Source: CAD feature listing. Evaluate the final solid. Frame: model axes, mm. Face numbers are marked on the shaded views. A direction names the side the tool comes from. Coordinates: 2 decimals unless noted, no trailing zeros. Write each loop counter-clockwise with the first axis right and the second up, starting at its lowest first coordinate (ties: lowest second). Pieces come first, ordered by that corner, then holes. Notation, with made-up numbers: (1, -21) -> (36, -21) arc R13 ccw to (36, -13) -> close; hole circle Ø6 at (-19.75, 83). An arc over 180 degrees is marked (long way). Write item = value, one per line.
from build123d import *

# Parameters (mm, degrees)
SKETCH_1_R          = 10
EXTRUDE_1_DEPTH     = 4
SKETCH_2_R          = 12
EXTRUDE_2_DEPTH     = 78
SKETCH_4_R          = 9
EXTRUDE_3_DEPTH     = 15
EXTRUDE_START       = -2
SKETCH_5_R          = 16
EXTRUDE_4_DEPTH     = 4
SKETCH_6_R          = 11
EXTRUDE_5_DEPTH     = 35
SKETCH_7_R          = 8
EXTRUDE_6_DEPTH     = 20
SKETCH_8_R          = 6
EXTRUDE_7_DEPTH     = 16
CUT_EXTRUDE_START   = 20
SKETCH_9_R          = 6
SKETCH_9_R_2        = 4
CUT_EXTRUDE_1_DEPTH = 2
CUT_EXTRUDE_START_2 = 8
CUT_EXTRUDE_2_DEPTH = 3


# Read off the part's stored shape, not the designer's step: M24 机械螺纹 螺柱1, M12 机械螺纹 螺柱1
with BuildPart() as part:
    # 草图1 → 凸台-拉伸1 (new body)
    with BuildSketch(Plane.XY):
        Circle(SKETCH_1_R)
    extrude(amount=EXTRUDE_1_DEPTH)

    # 草图2 → 凸台-拉伸2 (add)
    with BuildSketch(Plane.XY.offset(4)):
        Circle(SKETCH_2_R)
    extrude(amount=EXTRUDE_2_DEPTH)

    # M24 机械螺纹 螺柱1 outline → M24 机械螺纹 螺柱1 (revolve, cut)
    with BuildSketch(Plane.XZ):
        Polygon((12, 5.624), (10.376, 4), (12, 4), align=None)
    revolve(axis=Axis((0, 0, 0), (0, 0, 1)), mode=Mode.SUBTRACT)

    # 草图4 → 凸台-拉伸3 (add)
    with BuildSketch(Plane.XY.offset(82)):
        Circle(SKETCH_4_R)
    extrude(amount=EXTRUDE_3_DEPTH)

    # 草图5 → 凸台-拉伸4 (add)
    with BuildSketch(Plane.XY.offset(97).offset(EXTRUDE_START)):
        Circle(SKETCH_5_R)
    extrude(amount=-EXTRUDE_4_DEPTH)

    # 草图6 → 凸台-拉伸5 (add)
    with BuildSketch(Plane.XY.offset(97)):
        Circle(SKETCH_6_R)
    extrude(amount=EXTRUDE_5_DEPTH)

    # 草图7 → 凸台-拉伸6 (add)
    with BuildSketch(Plane.XY.offset(132)):
        Circle(SKETCH_7_R)
    extrude(amount=EXTRUDE_6_DEPTH)

    # 草图8 → 凸台-拉伸7 (add)
    with BuildSketch(Plane.XY.offset(152)):
        Circle(SKETCH_8_R)
    extrude(amount=EXTRUDE_7_DEPTH)

    # 草图9 → 切除-拉伸1 (cut)
    with BuildSketch(Plane.XY.offset(132).offset(CUT_EXTRUDE_START)):
        Circle(SKETCH_9_R)
        Circle(SKETCH_9_R_2, mode=Mode.SUBTRACT)
    extrude(amount=CUT_EXTRUDE_1_DEPTH, mode=Mode.SUBTRACT)

    # M12 机械螺纹 螺柱1 outline → M12 机械螺纹 螺柱1 (revolve, cut)
    with BuildSketch(Plane.XZ):
        Polygon((6, 168), (5.053, 168), (6, 167.053), align=None)
    revolve(axis=Axis((0, 0, 0), (0, 0, 1)), mode=Mode.SUBTRACT)

    # 草图11 → 切除-拉伸2 (cut)
    with BuildSketch(Plane(origin=(0, 0, 0), x_dir=(1, 0, 0), z_dir=(0, 1, 0)).offset(CUT_EXTRUDE_START_2)):
        with BuildLine():
            Line((-2.5, -147.5), (-2.5, -136.5))
            ThreePointArc((-2.5, -136.5), (0, -134), (2.5, -136.5))
            Line((2.5, -136.5), (2.5, -147.5))
            ThreePointArc((2.5, -147.5), (0, -150), (-2.5, -147.5))
        make_face()
    extrude(amount=-CUT_EXTRUDE_2_DEPTH, mode=Mode.SUBTRACT)


solid = part.part
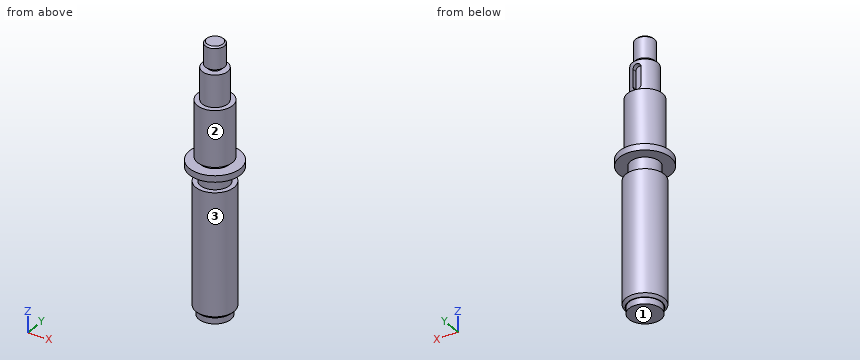
1) Cut plane A-A, the plane z = 70. Output: boundary loops of the cut face in (x, y).
Answer block:
outline = circle Ø24 at (0, 0)
2) Material intervals for probe 1 along Z at (x, y) = (10, -3.5); probe 2 along Z at (x, y) = (-1.5, -5.5); probe 3 along Z at (x, y) = (-10.5, 0.5), sorted ascending. Write a range as [from, to].
Answer block:
probe_1 = [4.22, 82], [91, 95], [97, 132]
probe_2 = [0, 152], [154, 167.35]
probe_3 = [4.14, 82], [91, 95], [97, 132]
3) First-contact query: pin 1 Ø12 at (x, z) = (7, 89.5) entering from +Y; pin 2 Ø8 at (x, y) = (-6.5, -12.5) entering from -Z; pin 3 Ø5 at (x, z) = (9, 79) entering from +Y. Flat tips, straight axial feed; report the tip coordinate or a pass-through.
Answer block:
pin_1 = 15.96
pin_2 = 4
pin_3 = 10.09
4) Reachability of the marked faces 1, 2 and 3 from +Z, -Z, +X, -X, +Y, -Y: full face, straight path, thin tool, end or side. Return the list, or none.
Answer block:
face_1 = -Z, +X, -X, +Y, -Y
face_2 = +Z
face_3 = -Z
